from build123d import *

# Parameters (mm, degrees)
SKETCH2_W           = 30
SKETCH2_H           = 50.1
SKETCH2_R           = 1.25
SKETCH2_R_2         = 5.5
BOSS_EXTRUDE1_DEPTH = 1.5
BOSS_EXTRUDE2_START = 15
SKETCH3_R           = 1.5
BOSS_EXTRUDE2_DEPTH = 1.5
BOSS_EXTRUDE3_START = -15
SKETCH3_2_R         = 1.5
BOSS_EXTRUDE3_DEPTH = 1.5


with BuildPart() as part:
    # Sketch2 → Boss-Extrude1 (new body)
    with BuildSketch(Plane(origin=(0, 0, 0), x_dir=(1, 0, 0), z_dir=(0, 1, 0))):
        with Locations((0, -0.55)):
            Rectangle(SKETCH2_W, SKETCH2_H)
        with Locations((-8, 12.5)):
            Circle(SKETCH2_R, mode=Mode.SUBTRACT)
        with Locations((-5.656854249, 18.156854249)):
            Circle(SKETCH2_R, mode=Mode.SUBTRACT)
        with Locations((0, 20.5)):
            Circle(SKETCH2_R, mode=Mode.SUBTRACT)
        with Locations((5.656854249, 18.156854249)):
            Circle(SKETCH2_R, mode=Mode.SUBTRACT)
        with Locations((8, 12.5)):
            Circle(SKETCH2_R, mode=Mode.SUBTRACT)
        with Locations((5.656854249, 6.843145751)):
            Circle(SKETCH2_R, mode=Mode.SUBTRACT)
        with Locations((0, 4.5)):
            Circle(SKETCH2_R, mode=Mode.SUBTRACT)
        with Locations((-5.656854249, 6.843145751)):
            Circle(SKETCH2_R, mode=Mode.SUBTRACT)
        with Locations((0, 12.5)):
            Circle(SKETCH2_R_2, mode=Mode.SUBTRACT)
    extrude(amount=BOSS_EXTRUDE1_DEPTH)

    # Sketch3 → Boss-Extrude2 (add)
    with BuildSketch(Plane(origin=(0, 0, 0), x_dir=(0, 0, -1), z_dir=(1, 0, 0)).offset(BOSS_EXTRUDE2_START)):
        with BuildLine():
            Line((24.5, 1.5), (18.69812916, 7.851243689))
            ThreePointArc((18.69812916, 7.851243689), (17.927938335, 8.404502374), (16.99999989, 8.6))
            Line((16.99999989, 8.6), (-21, 8.6))
            Line((-21, 8.6), (-21, 12.8))
            ThreePointArc((-21, 12.8), (-23.3, 15.1), (-25.6, 12.8))
            Line((-25.6, 12.8), (-25.6, 1.5))
            Line((-25.6, 1.5), (-25.6, 0))
            Line((-25.6, 0), (24.5, 0))
            Line((24.5, 0), (24.5, 1.5))
        make_face()
        with Locations((-23.3, 12.8)):
            Circle(SKETCH3_R, mode=Mode.SUBTRACT)
        with Locations((-17.00000011, 6.3)):
            Circle(SKETCH3_R, mode=Mode.SUBTRACT)
        with Locations((-1.1e-07, 6.3)):
            Circle(SKETCH3_R, mode=Mode.SUBTRACT)
        with Locations((16.99999989, 6.3)):
            Circle(SKETCH3_R, mode=Mode.SUBTRACT)
    extrude(amount=BOSS_EXTRUDE2_DEPTH)

    # Sketch3<2> → Boss-Extrude3 (add)
    with BuildSketch(Plane(origin=(0, 0, 0), x_dir=(0, 0, -1), z_dir=(1, 0, 0)).offset(BOSS_EXTRUDE3_START)):
        with BuildLine():
            Line((24.5, 1.5), (18.69812916, 7.851243689))
            ThreePointArc((18.69812916, 7.851243689), (17.927938335, 8.404502374), (16.99999989, 8.6))
            Line((16.99999989, 8.6), (-21, 8.6))
            Line((-21, 8.6), (-21, 12.8))
            ThreePointArc((-21, 12.8), (-23.3, 15.1), (-25.6, 12.8))
            Line((-25.6, 12.8), (-25.6, 1.5))
            Line((-25.6, 1.5), (-25.6, 0))
            Line((-25.6, 0), (24.5, 0))
            Line((24.5, 0), (24.5, 1.5))
        make_face()
        with Locations((-23.3, 12.8)):
            Circle(SKETCH3_2_R, mode=Mode.SUBTRACT)
        with Locations((-17.00000011, 6.3)):
            Circle(SKETCH3_2_R, mode=Mode.SUBTRACT)
        with Locations((-1.1e-07, 6.3)):
            Circle(SKETCH3_2_R, mode=Mode.SUBTRACT)
        with Locations((16.99999989, 6.3)):
            Circle(SKETCH3_2_R, mode=Mode.SUBTRACT)
    extrude(amount=-BOSS_EXTRUDE3_DEPTH)


solid = part.part
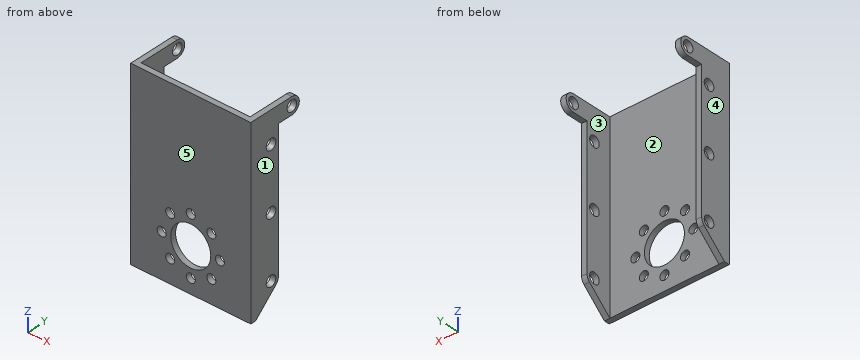
Build history of the part. All positions in model axes, mm. Face numbers are marked on the shaded views. A direction names the side the tool comes from. Coordinates: 2 decimals unless noted, no trailing zeros. Write each loop counter-clockwise with the first axis right and the second up, starting at its lowest first coordinate (ties: lowest second). Pieces come first, ordered by that corner, then holes.
(1) Cut at B-B on x = 0. List the corners of the cut face in (y, z).
(2) Cut at C-C on y = 9.5. List the corners of the cut face in (x, z).
(3) Pin check, flat tips, straight feed: pin 1 Ø4 at (x, z) = (5.5, -11) entering from +Y; pin 2 Ø3.5 at (y, z) = (12.8, 23.3) entering from -X; pin 3 Ø1.6 at (x, y) = (-15.5, 10) entering from -Z. Stop position of each tip, or through.
(4) Mould opens along X. For the marked faces 3, 4 and 5 say: pulls with the +X half, pulls with the -X half, needs draft (parallel to the pull), parting line crosses it, or undercut.
(5) 3-axis set-ups, long thin cutter, end or side, ignore diameter. For the marked faces 1 and 2: which of +Z, -Z, +X, -X, +Y, -Y reach the whole face in a straight line?
(6) Cut at A-A on z = -4.5. List the corners of the cut face in (x, y).
(7) Cut at D-D on z = 23.3. List the corners of the cut face in (x, y), and give its area (3 significant figures).
(8) Drill centre lines: line 1 (Z direction, x = 0, y = 0.55); line 2 (X direction, y = 7.75, z = 23); line 3 (Y direction, x = -15.95, z = 0). Where is each one in solid material? Low to high.
Working result:
1. outline: (0, -24.5) - (1.5, -24.5) - (1.5, -21.75) - (0, -21.75) - close; (0, -19.25) - (1.5, -19.25) - (1.5, -18) - (0, -18) - close; (0, -7) - (1.5, -7) - (1.5, -5.75) - (0, -5.75) - close; (0, -3.25) - (1.5, -3.25) - (1.5, 25.6) - (0, 25.6) - close
2. outline: (-16.5, 21) - (-15, 21) - (-15, 25.6) - (-16.5, 25.6) - close; (15, 21) - (16.5, 21) - (16.5, 25.6) - (15, 25.6) - close
3. pin 1: stops at y = 1.5
3. pin 2: stops at x = -16.5
3. pin 3: stops at z = 21
4. face 3: undercut
4. face 4: pulls with the -X half
4. face 5: needs draft
5. face 1: +Z, -Z, +X, +Y, -Y
5. face 2: +Z, -Z, +Y
6. outline: (-16.5, 0) - (-1.25, 0) - (-1.25, 1.5) - (-15, 1.5) - (-15, 8.6) - (-16.5, 8.6) - close; (1.25, 0) - (16.5, 0) - (16.5, 8.6) - (15, 8.6) - (15, 1.5) - (1.25, 1.5) - close
7. outline: (-16.5, 0) - (16.5, 0) - (16.5, 11.3) - (15, 11.3) - (15, 1.5) - (-15, 1.5) - (-15, 11.3) - (-16.5, 11.3) - close; (-16.5, 14.3) - (-15, 14.3) - (-15, 15.1) - (-16.5, 15.1) - close; (15, 14.3) - (16.5, 14.3) - (16.5, 15.1) - (15, 15.1) - close
7. area: 81.3 mm2
8. line 1: z = -24.5 to -21.75, -19.25 to -18, -7 to -5.75, -3.25 to 25.6
8. line 2: x = -16.5 to -15, 15 to 16.5
8. line 3: y = 0 to 4.8, 7.8 to 8.6
